from build123d import *

# Parameters (mm, degrees)
SKETCH1_R           = 20
BOSS_EXTRUDE1_DEPTH = 75
SKETCH2_R           = 10
CUT_EXTRUDE1_DEPTH  = 10
SKETCH3_R           = 2.5
CUT_EXTRUDE2_DEPTH  = 20
FILLET1_R           = 1


with BuildPart() as part:
    # Sketch1 → Boss-Extrude1 (new body)
    with BuildSketch(Plane.XY):
        Circle(SKETCH1_R)
    extrude(amount=BOSS_EXTRUDE1_DEPTH)

    # Sketch2 → Cut-Extrude1 (cut)
    with BuildSketch(Plane(origin=(20, 0, 0), x_dir=(0, 0, -1), z_dir=(1, 0, 0))):
        with Locations((-50, 0)):
            Circle(SKETCH2_R)
    extrude(amount=-CUT_EXTRUDE1_DEPTH, mode=Mode.SUBTRACT)

    # Sketch3 → Cut-Extrude2 (cut)
    with BuildSketch(Plane(origin=(20, 0, 0), x_dir=(0, 0, -1), z_dir=(1, 0, 0))):
        with Locations((-50, 0)):
            Circle(SKETCH3_R)
    extrude(amount=-CUT_EXTRUDE2_DEPTH, mode=Mode.SUBTRACT)

    # Fillet1
    fillet1_edges = [part.edges().sort_by_distance(p)[0] for p in [
        (10, 0, 52.5),
        (0, 0, 52.5),
        (17.320510975, 9.999994979, 50.010021457),
        (10, 0, 60),
    ]]
    fillet(fillet1_edges, radius=FILLET1_R - 0.0001)  # a hair under: the kernel refuses the full size


solid = part.part
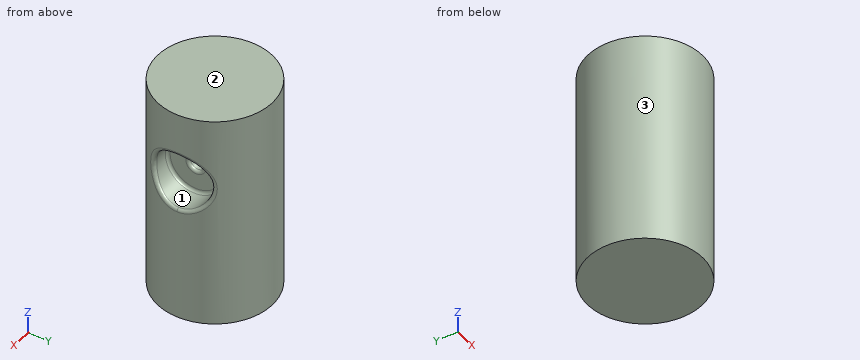
Part model, mm, in its own coordinate system. Face numbers are marked on the shaded views. Round coordinates to 2 decimals unless told otherwise and drop trailing zeros. Loops run counter-clockwise (first coordinate to the right, second up) from the corner with the lowest first, then second, coordinate; pieces in that order, holes last. Notation, with made-up numbers: (37.5, 61.5) - (53.5, 61.5) arc R27 cw to (53.5, 80.5) - close; hole circle Ø6 at (0, 38). An arc over 180 degrees is marked (long way). Answer as a JSON object with one key per item and string values.
Item 1: Pin check, flat tips, straight feed: pin 1 (1.5 mm diameter, centred on y = 1.5, z = 13, fed in from +X); pin 2 (0.9 mm diameter, centred on y = -0.5, z = 49.5, fed in from +X); pin 3 (10 mm diameter, centred on x = -5.5, y = 14.5, fed in from -Z); pin 4 (8 mm diameter, centred on y = 12, z = 63.5, fed in from -X). Stop position of each tip, or through.
Output:
{"pin 1": "x = 19.99", "pin 2": "x = 0", "pin 3": "z = 0", "pin 4": "x = -18.33"}
Item 2: Wall check: L1, parallel to X at y = -0.5, z = 22; L2, parallel to Y at x = 3, z = 50; L3, parallel to Y at x = 15, z = 55. Give the ranges that are in metal, low to high.
Output:
{"L1": "-19.99 to 19.99", "L2": "-19.77 to -2.5, 2.5 to 19.77", "L3": "-13.23 to -8.66, 8.66 to 13.23"}
Item 3: Band-saw the part on D-D on y = 12.5. List the corners of the cut face in (x, z).
Output:
{"outline": "(-15.61, 0) - (15.61, 0) - (15.61, 75) - (-15.61, 75) - close"}
Item 4: Band-saw the part on A-A on x = 12. List the corners of the cut face in (y, z).
Output:
{"outline": "(-16, 0) - (16, 0) - (16, 75) - (-16, 75) - close; hole circle Ø20 at (0, 50)"}
Item 5: Band-saw the part on C-C on x = -10. List the corners of the cut face in (y, z).
Output:
{"outline": "(-17.32, 0) - (17.32, 0) - (17.32, 75) - (-17.32, 75) - close"}
Item 6: Band-saw the part on B-B on z = 29. List the corners of the cut face in (x, y), plus the area to 3 significant figures.
Output:
{"outline": "circle Ø40 at (0, 0)", "area": "1,260 mm2"}
Item 7: Pull direction Y, two halves, no side cores. Call the marked faces 1, 2 and 3: pulls with the +Y half, pulls with the -Y half, needs draft (parallel to the pull), parting line crosses it, or undercut.
Output:
{"face 1": "undercut", "face 2": "needs draft", "face 3": "parting line crosses it"}
